Check sheet for the drawn part. Datum: minimum x, y, z corner. Units: mm. A direction names the side the tool comes from. Give positions to 0.01 mm unless a question says otherwise; leave off trailing zeros. Loops run counter-clockwise (first coordinate to the right, second up) from the corner with the lowest first, then second, coordinate; pieces in that order, holes last. Notation, with made-up numbers: (-8.75, 57.25) - (22.25, 57.25) arc R21 cw to (22.25, 68.25) - close; hole circle Ø2 at (61, -30). An arc over 180 degrees is marked (long way). Use one line per item in the form item = value.
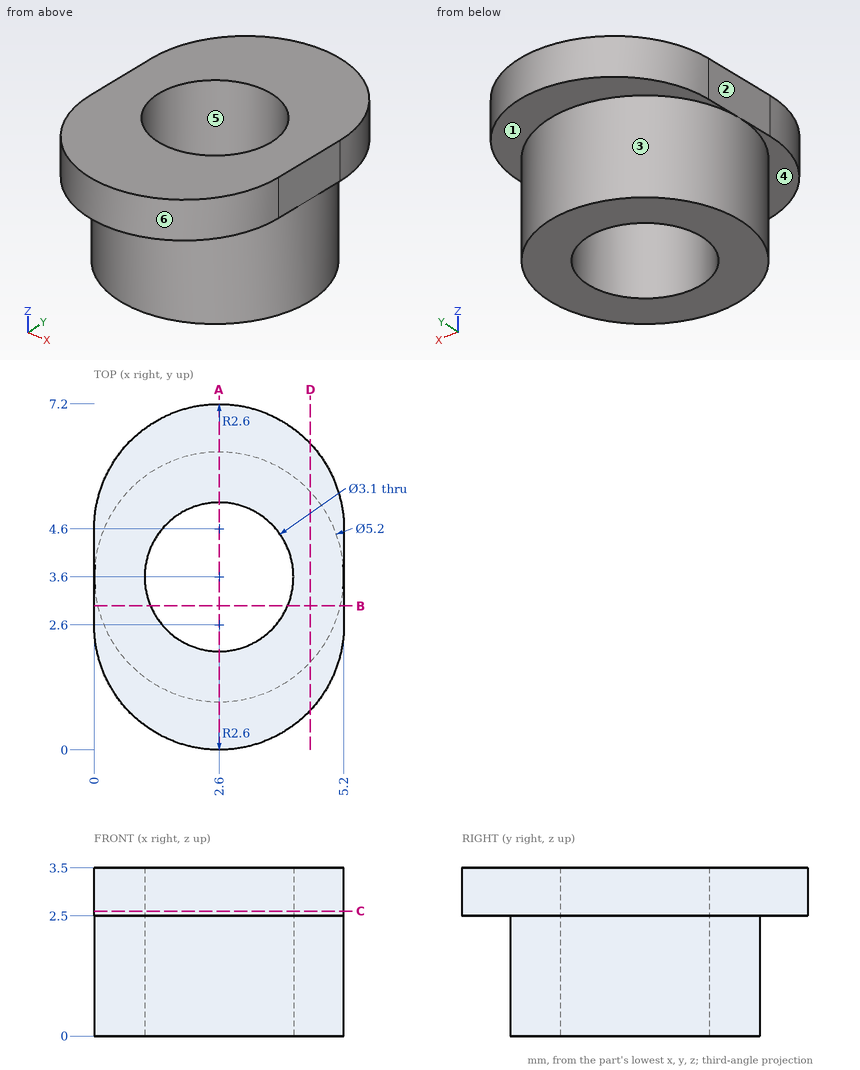
1. Scan lines: probe 1 along Y at (x, z) = (2.6, 1.55); probe 2 along Z at (x, y) = (4.45, 5.75); probe 3 along X at (y, z) = (4.5, 1.3). Record each from-to range of solid material in increasing order.
Result set:
probe_1 = 1 to 2.05, 5.15 to 6.2
probe_2 = 2.5 to 3.5
probe_3 = 0.16 to 1.34, 3.86 to 5.04
2. Draft check along Y on the marked faces 4, 5 and 6. Enter one of: released by +Y, released by -Y, zero draft, split by the parting line, or undercut.
Result set:
face_4 = zero draft
face_5 = undercut
face_6 = released by -Y
3. Section check D-D, the plane x = 4.5. Record the cut outline in (y, z), then the cut area to 3 significant figures.
Result set:
outline = (0.83, 2.5) - (1.83, 2.5) - (1.83, 0) - (5.37, 0) - (5.37, 2.5) - (6.37, 2.5) - (6.37, 3.5) - (0.83, 3.5) - close
area = 14.4 mm²
4. Tool access check on the marked faces 1, 2 and 3. Record the directions out of +Z, -Z, +X, -X, +Y, -Y that give a thin tool (end or side, any length) a straight path to the whole face; none if there is none.
Result set:
face_1 = -Z, +Y
face_2 = +Z, -Z, -X, +Y, -Y
face_3 = -Z
5. Section check C-C, the plane z = 2.6. Record the cut outline in (x, y), then the cut area to 3 significant figures.
Result set:
outline = (0, 2.6) arc R2.6 ccw to (5.2, 2.6) - (5.2, 4.6) arc R2.6 ccw to (0, 4.6) - close; hole circle Ø3.1 at (2.6, 3.6)
area = 24.1 mm²
6. Depth check by flat-ended pin: pin 1 Ø2 at (y, z) = (1, 2) entering from +X. Enter the tip coordinate at first touch or a pass-through.
Result set:
pin_1 = 5.09
7. Section check A-A, the plane x = 2.6. Record the cut outline in (y, z).
Result set:
outline = (0, 2.5) - (1, 2.5) - (1, 0) - (2.05, 0) - (2.05, 3.5) - (0, 3.5) - close; (5.15, 0) - (6.2, 0) - (6.2, 2.5) - (7.2, 2.5) - (7.2, 3.5) - (5.15, 3.5) - close
8. Section check B-B, the plane y = 3. Record the cut outline in (x, z), then the cut area to 4 significant figures.
Result set:
outline = (0, 2.5) - (0.07, 2.5) - (0.07, 0) - (1.17, 0) - (1.17, 3.5) - (0, 3.5) - close; (4.03, 0) - (5.13, 0) - (5.13, 2.5) - (5.2, 2.5) - (5.2, 3.5) - (4.03, 3.5) - close
area = 7.845 mm²
